Part model, mm, in its own coordinate system. A direction names the side the tool comes from. Round coordinates to 2 decimals unless told otherwise and drop trailing zeros. Loops run counter-clockwise (first coordinate to the right, second up) from the corner with the lowest first, then second, coordinate; pieces in that order, holes last. Notation, with made-up numbers: (-29, -10) -> (14, -10) arc R19 cw to (14, 12) -> close; hole circle Ø2 at (2.25, 42). An arc over 180 degrees is marked (long way). Use a Markdown table: item, result. Add a question column.
Item 1: Cut at B-B, the plane x = 35. List the corners of the cut face in (y, z).
Item 2: Cut at C-C, the plane z = 31. List the corners of the cut face in (x, y).
Item 3: Probe line 1 (Z direction, x = 17.5, y = -22.5); line 2 (X direction, y = -21.5, z = 3); line 3 (Y direction, x = 37, z = 29). List the from-to ranges inside material, lowest first. Write a range as [from, to].
Item 4: Flat gauge pins, fed straight in: pin 1 (12 mm diameter, centred on x = 4, y = -22, fed in from -Z); pin 2 (1 mm diameter, centred on y = -17.5, z = 32.5, fed in from +X); pin 3 (12 mm diameter, centred on x = 29.5, z = 7.5, fed in from +Y) (3 decimals); pin 4 (6 mm diameter, centred on x = 29, y = -23.5, fed in from -Z). Where does each tip first touch, or does it go through?
Item 5: Which spindle directions (+Z, -Z, +X, -X, +Y, -Y) get a long thin tool onto all of the face, cutting with end or side? Do faces 1 (the face through (20, -20, 60)), 2 (the face through (10, -8, 11)). Say none if no direction does.
Item 6: Cut at A-A, the plane y = -12. List the corners of the cut face in (x, z).
Item 7: Cut at D-D, the plane y = -5.5. List the corners of the cut face in (x, z), plus the area to 3 significant figures.
```python
from build123d import *

# Parameters (mm, degrees)
SKETCH_2_W          = 60
SKETCH_2_H          = 40
EXTRUDE_1_DEPTH     = 40
CUT_EXTRUDE_1_DEPTH = 40
EXTRUDE_2_REACH     = 84.462
SKETCH_7_W          = 10
SKETCH_7_H          = 40


with BuildPart() as part:
    # 草圖2 → 填料-伸長1 (new body)
    with BuildSketch(Plane(origin=(0, 0, 0), x_dir=(0, 0, -1), z_dir=(1, 0, 0))):
        with Locations((-30, -20)):
            Rectangle(SKETCH_2_W, SKETCH_2_H)
    extrude(amount=EXTRUDE_1_DEPTH)

    # 草圖3 → 除料-伸長1 (cut)
    with BuildSketch(Plane(origin=(0, 0, 0), x_dir=(1, 0, 0), z_dir=(0, 1, 0))):
        Polygon((30, 0), (40, -40), (40, 0), align=None)
    extrude(amount=-CUT_EXTRUDE_1_DEPTH, mode=Mode.SUBTRACT)

    # 除料-掃出1: sweep along a path in 草圖6
    with BuildLine(Plane(origin=(28.235294118, 0, -7.058823529), x_dir=(-0.24253562503633305, 0, -0.9701425001453319), z_dir=(0.9701425001453319, 0, -0.24253562503633305))) as sweep_1_path:
        Line((-48.507125007, 0), (-7.276068751, -30))
    # 草圖5 → 除料-掃出1 (sweep, cut)
    with BuildSketch(Plane(origin=(0, 0, 0), x_dir=(1, 0, 0), z_dir=(0, 1, 0))):
        Polygon((30, 0), (10, 0), (10, -40), (40, -40), align=None)
    sweep(path=sweep_1_path.line, mode=Mode.SUBTRACT)

    # 填料-伸長2: up to this face of the body (flat: up to its plane)
    extrude_2_end = Plane(part.part.faces().sort_by_distance((20, -15, 20))[0])
    # 草圖7 → 填料-伸長2 (add, up to the picked face)
    with BuildSketch(Plane(origin=(0, 0, 0), x_dir=(1, 0, 0), z_dir=(0, 1, 0)), mode=Mode.PRIVATE) as extrude_2_sk1:
        with Locations((5, -20)):
            Rectangle(SKETCH_7_W, SKETCH_7_H)
    extrude_2_tool1 = split(extrude(extrude_2_sk1.sketch, amount=-EXTRUDE_2_REACH, mode=Mode.PRIVATE), bisect_by=extrude_2_end, keep=Keep.BOTH, mode=Mode.PRIVATE)
    add(extrude_2_tool1.solids().sort_by(Axis((5, 0, 20), (0, -1, 0)))[0])


solid = part.part
```
A:
| question | item | result |
|---|---|---|
| 1 | outline | (-40, 20) -> (-15, 20) -> (0, 40) -> (0, 60) -> (-40, 60) -> close |
| 2 | outline | (0, -40) -> (37.75, -40) -> (37.75, -6.75) -> (10, -6.75) -> (10, 0) -> (0, 0) -> close |
| 3 | line 1 | z = [10, 60] |
| 3 | line 2 | x = [0, 10] |
| 3 | line 3 | y = [-40, -8.25] |
| 4 | pin 1 | stops at z = 0 |
| 4 | pin 2 | stops at x = 38.25 |
| 4 | pin 3 | stops at y = -19.875 |
| 4 | pin 4 | stops at z = 4.67 |
| 5 | face 1 | +Z, +X, -X, +Y, -Y |
| 5 | face 2 | -Z, +X, +Y |
| 6 | outline | (0, 0) -> (10, 0) -> (10, 24) -> (36, 24) -> (40, 40) -> (40, 60) -> (0, 60) -> close |
| 7 | outline | (0, 0) -> (10, 0) -> (10, 32.67) -> (38.17, 32.67) -> (40, 40) -> (40, 60) -> (0, 60) -> close |
| 7 | area | 1,410 mm^2 |
